Build history of the part. All positions in model axes, mm. A direction names the side the tool comes from. Give positions to 0.01 mm unless a question says otherwise; leave off trailing zeros. Loops run counter-clockwise (first coordinate to the right, second up) from the corner with the lowest first, then second, coordinate; pieces in that order, holes last. Notation, with made-up numbers: (82, 22.5) -> (123, 22.5) arc R26 cw to (123, 51.5) -> close; hole circle Ø7 at (-13, 1). An arc over 180 degrees is marked (long way). Answer as a JSON object with one key per item and string values. Group by question number.
Q1. Tool access for faces 4 (the flat face through (-15, 197, 0)), 5 (the flat face through (-20, 197, -8)): list every direction of +Z, -Z, +X, -X, +Y, -Y with a clear straight run to the whole face (end or side of a thin tool).
Q2. Band-saw the part on A-A, the plane z = 0.25. Write the cut outline in (x, y).
Q3. Band-saw the part on C-C, the plane y = 93. Write the cut outline in (x, z), plus the area to 3 significant figures.
Q4. Wall check: probe 1 along Y at (x, z) = (0, -4.5); probe 2 along Z at (x, y) = (-18, 74); probe 3 along X at (y, z) = (0, 4.5). Give the ranges that are in metal, low to high. Write a range as from..to.
Q5. Two-plate mould, pull along Z, no slides. Class faces 1 (the flat face through (15, 197, 0)), 2 (the flat face through (0, 197, -12)), 3 (the flat face through (20, 197, -8)): pulls with the +Z half, pulls with the -Z half, needs draft (parallel to the pull), parting line crosses it, or undercut.
Q6. Drop flat-ended pins along their axis: pin 1 (2.5 mm diameter, centred on y = 121.5, z = 1, fed in from -X); pin 2 (21 mm diameter, centred on x = 0, y = 0, fed in from -Z); pin 3 (12 mm diameter, centred on x = -3, z = -1.5, fed in from +Y). Give the stop position or say it passes through.
Q7. Band-saw the part on B-B, the plane x = 0. Write the cut outline in (y, z).
from build123d import *
from build123d.topology import SkipClean

# Parameters (mm, degrees)
BOSS_EXTRUDE1_DEPTH = 400
BOSS_EXTRUDE2_REACH = 403.218
SKETCH2_R           = 20
FILLET1_R           = 10
CUT_EXTRUDE1_REACH  = 423.16
SKETCH3_R           = 13


with BuildPart() as part:
    # Sketch1 → Boss-Extrude1 (new body)
    with BuildSketch(Plane(origin=(0, 0, 0), x_dir=(1, 0, 0), z_dir=(0, 1, 0))):
        Polygon((-20, 12), (20, 12), (20, 4), (15, 4), (15, -4), (20, -4), (20, -12), (-20, -12), (-20, -4), (-15, -4), (-15, 4), (-20, 4), align=None)
    extrude(amount=BOSS_EXTRUDE1_DEPTH)

    # Boss-Extrude2: up to this face of the body (flat: up to its plane)
    boss_extrude2_end = Plane(part.part.faces().sort_by_distance((0, 200, 12))[0])
    # Sketch2 → Boss-Extrude2 (add, up to the picked face)
    with BuildSketch(Plane(origin=(0, 0, -12), x_dir=(-1, 0, 0), z_dir=(0, 0, -1)), mode=Mode.PRIVATE) as boss_extrude2_sk1:
        Circle(SKETCH2_R)
    boss_extrude2_tool1 = split(extrude(boss_extrude2_sk1.sketch, amount=-BOSS_EXTRUDE2_REACH, mode=Mode.PRIVATE), bisect_by=boss_extrude2_end, keep=Keep.BOTH, mode=Mode.PRIVATE)
    boss_extrude2 = boss_extrude2_tool1.solids().sort_by(Axis((0, 0, -12), (0, 0, 1)))[0]
    add(boss_extrude2)

    # Mirror1: Boss-Extrude2 across plane
    with SkipClean():  # the faces are left unmerged after this step: merging them gives an invalid solid
        add(boss_extrude2.mirror(Plane.ZX.offset(200)))
    add(part.part.scale(1), mode=Mode.REPLACE)  # the faces are merged on a copy

    # Fillet1
    fillet1_edges = [part.edges().sort_by_distance(p)[0] for p in [
        (15, 13.228756555, 0),
        (-15, 13.228756555, 0),
        (-15, 386.771243445, 0),
        (15, 386.771243445, 0),
    ]]
    fillet(fillet1_edges, radius=FILLET1_R)

    # Sketch3 → Cut-Extrude1 (cut, up to next)
    with BuildSketch(Plane(origin=(0, 0, -12), x_dir=(-1, 0, 0), z_dir=(0, 0, -1)), mode=Mode.PRIVATE) as cut_extrude1_sk1:
        with Locations((0, 400)):
            Circle(SKETCH3_R)
    cut_extrude1_tool1 = extrude(cut_extrude1_sk1.sketch, amount=-CUT_EXTRUDE1_REACH, mode=Mode.PRIVATE) & part.part
    cut_extrude1 = cut_extrude1_tool1.solids().sort_by_distance((0, 400, -12))[0]
    add(cut_extrude1, mode=Mode.SUBTRACT)

    # Mirror2: Cut-Extrude1 across plane
    add(cut_extrude1.mirror(Plane.ZX.offset(200)), mode=Mode.SUBTRACT)


solid = part.part
Worked answers:
{
 "1": {"face 4": "-X", "face 5": "+Z, -Z, -X, +Y, -Y"},
 "2": {"outline": "(-16.67, 11.06) arc R20 ccw (long way) to (16.67, 11.06) arc R10 cw to (15, 16.58) -> (15, 383.42) arc R10 cw to (16.67, 388.94) arc R20 ccw (long way) to (-16.67, 388.94) arc R10 cw to (-15, 383.42) -> (-15, 16.58) arc R10 cw to start; hole circle Ø26 at (0, 0); hole circle Ø26 at (0, 400)"},
 "3": {"outline": "(-20, -12) -> (20, -12) -> (20, -4) -> (15, -4) -> (15, 4) -> (20, 4) -> (20, 12) -> (-20, 12) -> (-20, 4) -> (-15, 4) -> (-15, -4) -> (-20, -4) -> close", "area": "880 mm2"},
 "4": {"probe 1": "-20..-13, 13..387, 413..420", "probe 2": "-12..-4, 4..12", "probe 3": "-20..-13, 13..20"},
 "5": {"face 1": "undercut", "face 2": "pulls with the -Z half", "face 3": "needs draft"},
 "6": {"pin 1": "x = -15", "pin 2": "through", "pin 3": "y = 420"},
 "7": {"outline": "(-20, -12) -> (-13, -12) -> (-13, 12) -> (-20, 12) -> close; (13, -12) -> (387, -12) -> (387, 12) -> (13, 12) -> close; (413, -12) -> (420, -12) -> (420, 12) -> (413, 12) -> close"}
}
